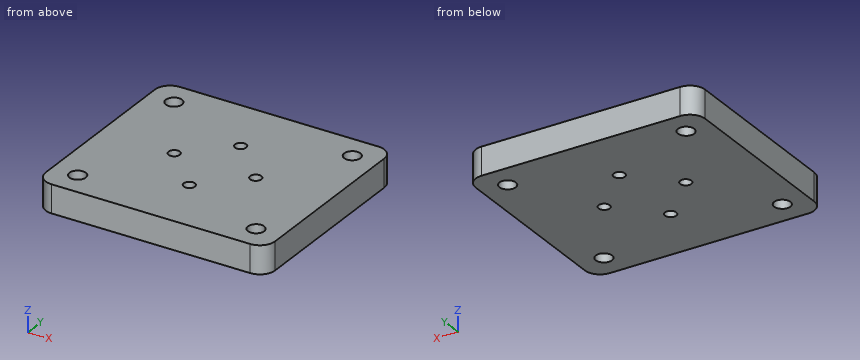
Solid Edge part; units mm, degrees
sketch "Sketch1" plane through (0, 0, 0) normal (0, 0, 1) x (1, 0, 0)
  line L0 (22.5, -20) -> (-22.5, -20)
  line L1 (-22.5, -20) -> (-22.5, 20)
  line L2 (-22.5, 20) -> (22.5, 20)
  line L3 (22.5, 20) -> (22.5, -20)
  dimension "D1" = 22.5
  dimension "D2" = 22.5
extrude "Protrusion1" add sketch "Sketch1" along normal blind 5.5
hole "Hole_1" at (0, -8, 5.5) direction (0, 0, -1) diameter 2.2 end up to next
hole "Hole1" at (8, 0, 5.5) direction (0, 0, -1) diameter 2.2 end up to next
hole "Hole2" at (-8, 0, 5.5) direction (0, 0, -1) diameter 2.2 end up to next
hole "Hole3" at (0, 8, 5.5) direction (0, 0, -1) diameter 2.2 end up to next
hole "Hole_5" at (-17.5, 15, 5.5) direction (0, 0, -1) diameter 3.2 end up to next
hole "Hole4" at (17.5, 15, 5.5) direction (0, 0, -1) diameter 3.2 end up to next
hole "Hole5" at (17.5, -15, 5.5) direction (0, 0, -1) diameter 3.2 end up to next
hole "Hole6" at (-17.5, -15, 5.5) direction (0, 0, -1) diameter 3.2 end up to next
fillet "Round_1" radius 3 4 edges at (22.5, -20, 2.75) (22.5, 20, 2.75) (-22.5, -20, 2.75) (-22.5, 20, 2.75)
properties material "木材, アッシュ"
Source: CAD feature listing. Evaluate the final solid. Frame: model axes, mm. Coordinates: 2 decimals unless noted, no trailing zeros. Write each loop counter-clockwise with the first axis right and the second up, starting at its lowest first coordinate (ties: lowest second). Pieces come first, ordered by that corner, then holes. Notation, with made-up numbers: M 74,-7 L 112,-7 A13 ccw 112,-3 Z; hole C -38.5,73.25 d2. An arc over 180 degrees is marked long. Use a Markdown table: item, result.
1) Section A-A, the plane x = -8. Output: boundary loops of the cut face in (y, z), then the cut area to 3 significant figures.
Conclusion:
| item | result |
|---|---|
| outline | M -20,0 L -1.1,0 L -1.1,5.5 L -20,5.5 Z; M 1.1,0 L 20,0 L 20,5.5 L 1.1,5.5 Z |
| area | 208 mm^2 |
2) Section C-C, the plane x = -17.5. Output: boundary loops of the cut face in (y, z).
Conclusion:
| item | result |
|---|---|
| outline | M -20,0 L -16.6,0 L -16.6,5.5 L -20,5.5 Z; M -13.4,0 L 13.4,0 L 13.4,5.5 L -13.4,5.5 Z; M 16.6,0 L 20,0 L 20,5.5 L 16.6,5.5 Z |
3) Section B-B, the plane y = 15. Output: boundary loops of the cut face in (x, z), then the cut area to 3 significant figures.
Conclusion:
| item | result |
|---|---|
| outline | M -22.5,0 L -19.1,0 L -19.1,5.5 L -22.5,5.5 Z; M -15.9,0 L 15.9,0 L 15.9,5.5 L -15.9,5.5 Z; M 19.1,0 L 22.5,0 L 22.5,5.5 L 19.1,5.5 Z |
| area | 212 mm^2 |
4) Ray query, L1, parallel to Y at x = -17.5, z = 1.9; L2, parallel to X at y = 0, z = 3.6; L3, parallel to Y at x = 18, z = 1. Return the intervals inside material, ascending.
Conclusion:
| item | result |
|---|---|
| L1 | y = -20 to -16.6, -13.4 to 13.4, 16.6 to 20 |
| L2 | x = -22.5 to -9.1, -6.9 to 6.9, 9.1 to 22.5 |
| L3 | y = -20 to -16.52, -13.48 to 13.48, 16.52 to 20 |
5) First-contact query: pin 1 Ø2.5 at (x, y) = (17.5, 15) entering from -Z. Flat tip, straight axial feed; report the tip coordinate or a pass-through.
Conclusion:
| item | result |
|---|---|
| pin 1 | passes through |
6) Section D-D, the plane y = -8. Output: boundary loops of the cut face in (x, z), then the cut area to 3 significant figures.
Conclusion:
| item | result |
|---|---|
| outline | M -22.5,0 L -1.1,0 L -1.1,5.5 L -22.5,5.5 Z; M 1.1,0 L 22.5,0 L 22.5,5.5 L 1.1,5.5 Z |
| area | 235 mm^2 |
